Build history of the part. All positions in model axes, mm. Coordinates: 2 decimals unless noted, no trailing zeros. Write each loop counter-clockwise with the first axis right and the second up, starting at its lowest first coordinate (ties: lowest second). Pieces come first, ordered by that corner, then holes.
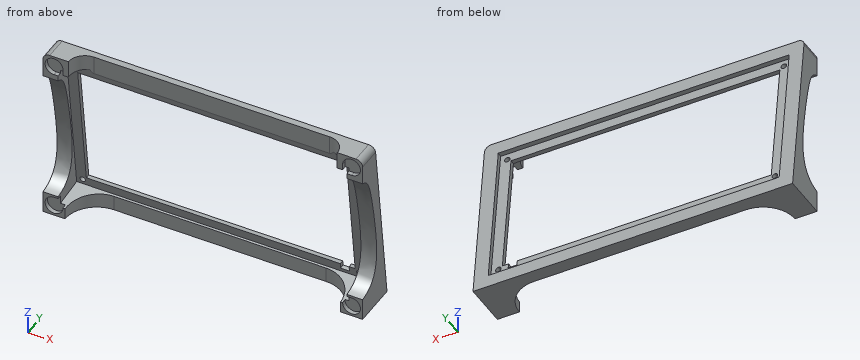
```python
from build123d import *

# Parameters (mm, degrees)
BOSS_EXTRUDE1_DEPTH       = 17.38
BOSS_EXTRUDE1_DEPTH_BACK  = 3
SKETCH1_W                 = 145
SKETCH1_H                 = 80.5
SKETCH1_W_2               = 132
SKETCH1_H_2               = 68.1
SKETCH2_W                 = 145.621836594
SKETCH2_H                 = 81.229894902
CUT_EXTRUDE1_DEPTH        = 10.38
FILLET1_R                 = 3
BOSS_EXTRUDE17_DEPTH      = 17.38
BOSS_EXTRUDE17_DEPTH_BACK = 3
SKETCH5_W                 = 132
SKETCH5_H                 = 68.1
SKETCH5_W_2               = 122
SKETCH5_H_2               = 58.53632086
SKETCH9_W                 = 144.471640976
SKETCH9_H                 = 84.136143584
CUT_EXTRUDE5_DEPTH        = 9.6
SKETCH6_W                 = 132
SKETCH6_H                 = 68.611419114
CUT_EXTRUDE6_DEPTH        = 2
CUT_EXTRUDE9_DEPTH        = 10.7
CUT_EXTRUDE12_START       = -145
CUT_EXTRUDE12_DEPTH       = 145
CUT_EXTRUDE13_DEPTH       = 10
SKETCH21_W                = 131
SKETCH21_H                = 67.1
CUT_EXTRUDE14_DEPTH       = 30
CUT_EXTRUDE15_START       = -2
CUT_EXTRUDE15_DEPTH       = 2
CUT_EXTRUDE17_DEPTH       = 10
CUT_EXTRUDE18_DEPTH       = 10


# Read off the part's stored shape, not the designer's step: Cut-Extrude12, Cut-Extrude15
with BuildPart() as part:
    # Sketch1 → Boss-Extrude1 (new, two sides: drawn at the far end of the back side and taken through both)
    with BuildSketch(Plane(origin=(0, 0, 0), x_dir=(1, 0, 0), z_dir=(0, 1, 0)).offset(-BOSS_EXTRUDE1_DEPTH_BACK)):
        Rectangle(SKETCH1_W, SKETCH1_H)
        Rectangle(SKETCH1_W_2, SKETCH1_H_2, mode=Mode.SUBTRACT)
    extrude(amount=BOSS_EXTRUDE1_DEPTH + BOSS_EXTRUDE1_DEPTH_BACK)

    # Sketch2 → Cut-Extrude1 (cut)
    with BuildSketch(Plane(origin=(0, 12.253191712, 1.504502764), x_dir=(-1, 0, 0), z_dir=(0, 0.9925461516413239, 0.12186934340513403))):
        with Locations((0.310918297, -1.453124341)):
            Rectangle(SKETCH2_W, SKETCH2_H)
    extrude(amount=CUT_EXTRUDE1_DEPTH, mode=Mode.SUBTRACT)

    # Fillet1
    fillet1_edges = [part.edges().sort_by_distance(p)[0] for p in [
        (72.5, 2.247921424, 40.25),
        (-72.5, 2.247921424, 40.25),
    ]]
    fillet(fillet1_edges, radius=FILLET1_R)

    # Sketch5 → Boss-Extrude17 (add, two sides: drawn at the far end of the back side and taken through both)
    with BuildSketch(Plane(origin=(0, 0, 0), x_dir=(1, 0, 0), z_dir=(0, 1, 0)).offset(-BOSS_EXTRUDE17_DEPTH_BACK)):
        Rectangle(SKETCH5_W, SKETCH5_H)
        Rectangle(SKETCH5_W_2, SKETCH5_H_2, mode=Mode.SUBTRACT)
    extrude(amount=BOSS_EXTRUDE17_DEPTH + BOSS_EXTRUDE17_DEPTH_BACK)

    # Sketch9 → Cut-Extrude5 (cut)
    with BuildSketch(Plane(origin=(0, 12.253191712, 1.504502764), x_dir=(1, 0, 0), z_dir=(0, 0.9925461516413238, 0.12186934340513406))):
        Rectangle(SKETCH9_W, SKETCH9_H)
    extrude(amount=CUT_EXTRUDE5_DEPTH, mode=Mode.SUBTRACT)

    # Sketch6 → Cut-Extrude6 (cut)
    with BuildSketch(Plane(origin=(0, 12.253191712, 1.504502764), x_dir=(-1, 0, 0), z_dir=(0, 0.9925461516413239, 0.12186934340513403))):
        with Locations((0, -1.515801317)):
            Rectangle(SKETCH6_W, SKETCH6_H)
    extrude(amount=-CUT_EXTRUDE6_DEPTH, mode=Mode.SUBTRACT)

    # Sketch12 → Cut-Extrude9 (cut)
    with BuildSketch(Plane(origin=(0, 0, -40.25), x_dir=(-1, 0, 0), z_dir=(0, 0, -1))):
        with BuildLine():
            Line((62.5, -3), (62.500586031, -3))
            ThreePointArc((62.500586031, -3), (58.288781544, 7.168195513), (48.120586031, 11.38))
            Line((48.120586031, 11.38), (0, 11.38))
            Line((0, 11.38), (-48.120586031, 11.38))
            ThreePointArc((-48.120586031, 11.38), (-58.288781544, 7.168195513), (-62.500586031, -3))
            Line((-62.500586031, -3), (62.5, -3))
        make_face()
    extrude(amount=-CUT_EXTRUDE9_DEPTH, mode=Mode.SUBTRACT)

    # Cut-Extrude12 outline → Cut-Extrude12 (cut)
    with BuildSketch(Plane.ZY.offset(72.5).offset(CUT_EXTRUDE12_START)):
        with BuildLine():
            Line((-30.25, -3), (28.75, -3))
            add(Edge.make_bspline(
                [(28.75, -3), (26.32968346, 4.271531969), (19.440941834, 4.451750453), (-1.874181617, 6.089281656), (-27.421780079, 18.432975247), (-30.25, -3)],
                knots=[0.042214979, 0.042214979, 0.042214979, 0.042214979, 0.042214979, 0.042214979, 1.042214979, 1.042214979, 1.042214979, 1.042214979, 1.042214979, 1.042214979], degree=5))
        make_face()
    extrude(amount=CUT_EXTRUDE12_DEPTH, mode=Mode.SUBTRACT)

    # Sketch19 → Cut-Extrude13 (cut)
    with BuildSketch(Plane(origin=(0, 10.268099409, 1.260764077), x_dir=(1, 0, 0), z_dir=(0, 0.9925461516413238, 0.12186934340513403))):
        with BuildLine():
            ThreePointArc((61.5, 32.0425), (61.866116524, 31.158616524), (62.75, 30.7925))
            Line((62.75, 30.7925), (62.75, 32.0425))
            Line((62.75, 32.0425), (61.5, 32.0425))
        make_face()
        with BuildLine():
            Line((62.75, 32.0425), (62.75, 30.7925))
            ThreePointArc((62.75, 30.7925), (63.633883476, 31.158616524), (64, 32.0425))
            ThreePointArc((64, 32.0425), (62.75, 33.2925), (61.5, 32.0425))
            Line((61.5, 32.0425), (62.75, 32.0425))
        make_face()
        with BuildLine():
            ThreePointArc((64, -29.5425), (63.633883476, -28.658616524), (62.75, -28.2925))
            Line((62.75, -28.2925), (62.75, -29.5425))
            Line((62.75, -29.5425), (61.5, -29.5425))
            ThreePointArc((61.5, -29.5425), (62.75, -30.7925), (64, -29.5425))
        make_face()
        with BuildLine():
            Line((62.75, -29.5425), (62.75, -28.2925))
            ThreePointArc((62.75, -28.2925), (61.866116524, -28.658616524), (61.5, -29.5425))
            Line((61.5, -29.5425), (62.75, -29.5425))
        make_face()
        with BuildLine():
            ThreePointArc((-61.5, -29.5425), (-61.866116524, -28.658616524), (-62.75, -28.2925))
            Line((-62.75, -28.2925), (-62.75, -29.5425))
            Line((-62.75, -29.5425), (-61.5, -29.5425))
        make_face()
        with BuildLine():
            Line((-62.75, -29.5425), (-62.75, -28.2925))
            ThreePointArc((-62.75, -28.2925), (-63.633883476, -30.426383476), (-61.5, -29.5425))
            Line((-61.5, -29.5425), (-62.75, -29.5425))
        make_face()
        with BuildLine():
            ThreePointArc((-61.5, 32.0425), (-63.633883476, 32.926383476), (-62.75, 30.7925))
            Line((-62.75, 30.7925), (-62.75, 32.0425))
            Line((-62.75, 32.0425), (-61.5, 32.0425))
        make_face()
        with BuildLine():
            Line((-62.75, 32.0425), (-62.75, 30.7925))
            ThreePointArc((-62.75, 30.7925), (-61.866116524, 31.158616524), (-61.5, 32.0425))
            Line((-61.5, 32.0425), (-62.75, 32.0425))
        make_face()
    extrude(amount=-CUT_EXTRUDE13_DEPTH, mode=Mode.SUBTRACT)

    # Sketch21 → Cut-Extrude14 (cut)
    with BuildSketch(Plane(origin=(0, 8.283007106, 1.01702539), x_dir=(1, 0, 0), z_dir=(0, 0.9925461516413238, 0.12186934340513403))):
        with Locations((-0.141032576, 0.996407471)):
            Rectangle(SKETCH21_W, SKETCH21_H)
    extrude(amount=-CUT_EXTRUDE14_DEPTH, mode=Mode.SUBTRACT)

    # Cut-Extrude15 outline → Cut-Extrude15 (cut)
    with BuildSketch(Plane(origin=(0, -3, 0), x_dir=(-1, 0, 0), z_dir=(0, -1, 0)).offset(CUT_EXTRUDE15_START)):
        with BuildLine():
            Line((67.499992595, -31.228634541), (63.449992595, -31.228634541))
            Line((63.449992595, -31.228634541), (63.449992595, -35.278634541))
            ThreePointArc((63.449992595, -35.278634541), (70.363775058, -38.142417005), (67.499992595, -31.228634541))
        make_face()
        with BuildLine():
            Line((63.449999996, 31.2), (67.499999996, 31.2))
            ThreePointArc((67.499999996, 31.2), (70.363782459, 38.113782464), (63.449999996, 35.25))
            Line((63.449999996, 35.25), (63.449999996, 31.2))
        make_face()
        with BuildLine():
            Line((-67.5, 31.2), (-63.45, 31.2))
            Line((-63.45, 31.2), (-63.45, 35.25))
            ThreePointArc((-63.45, 35.25), (-70.363782464, 38.113782464), (-67.5, 31.2))
        make_face()
        with BuildLine():
            Line((-63.45, -31.2), (-67.5, -31.2))
            ThreePointArc((-67.5, -31.2), (-70.363782464, -38.113782464), (-63.45, -35.25))
            Line((-63.45, -35.25), (-63.45, -31.2))
        make_face()
    extrude(amount=CUT_EXTRUDE15_DEPTH, mode=Mode.SUBTRACT)

    # Sketch25 → Cut-Extrude17 (cut)
    with BuildSketch(Plane(origin=(0, 8.283007106, 1.01702539), x_dir=(1, 0, 0), z_dir=(0, -0.9925461516413238, -0.1218693434051341))):
        Polygon((58.22, -33.01262228), (58.22, -32.0425), (58.22, -30.51262228), (54.22, -30.51262228), (54.22, -33.01262228), align=None)
    extrude(amount=-CUT_EXTRUDE17_DEPTH, mode=Mode.SUBTRACT)

    # Sketch26 → Cut-Extrude18 (cut)
    with BuildSketch(Plane.XY.offset(40.25)):
        with BuildLine():
            ThreePointArc((-53.509718644, 4.495842847), (-58.810079952, 2.300361308), (-61.005561492, -3))
            Line((-61.005561492, -3), (-61, -3))
            Line((-61, -3), (59.5, -3))
            Line((59.5, -3), (61.005561492, -3))
            ThreePointArc((61.005561492, -3), (58.810079952, 2.300361308), (53.509718644, 4.495842847))
            Line((53.509718644, 4.495842847), (53.241634956, 4.495842847))
            Line((53.241634956, 4.495842847), (0, 4.495842847))
            Line((0, 4.495842847), (-53.509718644, 4.495842847))
        make_face()
    extrude(amount=-CUT_EXTRUDE18_DEPTH, mode=Mode.SUBTRACT)


solid = part.part
```
1. Probe line 1 along X through (y, z) = (-2.25, -35.25); line 2 along X through (y, z) = (-2.4, 35.25); line 3 along X through (y, z) = (11, -28). List the from-to ranges inside material, lowest first.
Computed values:
line 1: x = -72.5 to -71.55, -63.45 to -62.48, 62.48 to 63.45, 71.55 to 72.5
line 2: x = -72.5 to -71.55, -63.45 to -60.98, 60.98 to 63.45, 71.55 to 72.5
line 3: x = -72.5 to -65.64, 65.36 to 72.5
2. Saw through at B-B on x = -50.5. List the corners of the cut face in (y, z), plus the area to 3 significant figures.
Computed values:
outline: (4.5, 31.86) - (4.81, 29.27) - (6.83, 29.27) - (6.27, 33.81) - (8.26, 34.05) - (7.5, 40.25) - (4.5, 40.25) - close; (11.18, -40.25) - (17.38, -40.25) - (16.62, -34.05) - (14.63, -34.29) - (14.02, -29.27) - (12, -29.27) - (12.49, -33.27) - (11.18, -33.43) - close
area: 77.0 mm2
3. Flat gauge pins, fed straight in: pin 1 (1 mm diameter, centred on x = 1.5, y = 5.5, fed in from -Z); pin 2 (0.6 mm diameter, centred on x = -22, y = 13.5, fed in from +Z); pin 3 (5.5 mm diameter, centred on x = 16.5, z = -36.5, fed in from -Y). Where does each tip first touch, or does it go through?
Computed values:
pin 1: stops at z = 29.27
pin 2: stops at z = -29.27
pin 3: stops at y = 11.38
4. Saw through at A-A on x = 6. List the corners of the cut face in (y, z).
Computed values:
outline: (4.5, 31.86) - (4.81, 29.27) - (6.83, 29.27) - (6.27, 33.81) - (8.26, 34.05) - (7.5, 40.25) - (4.5, 40.25) - close; (11.38, -40.25) - (17.38, -40.25) - (16.62, -34.05) - (14.63, -34.29) - (14.02, -29.27) - (12, -29.27) - (12.49, -33.27) - (11.38, -33.41) - close
